Build history of the part. All positions in model axes, mm. A direction names the side the tool comes from. Round coordinates to 2 decimals unless told otherwise and drop trailing zeros. Loops run counter-clockwise (first coordinate to the right, second up) from the corner with the lowest first, then second, coordinate; pieces in that order, holes last. Notation, with made-up numbers: M 3,46.25 L 16,46.25 A15 ccw 16,55.25 Z; hole C 57,9 d3. An arc over 180 degrees is marked long. One line per item, written item: value.
```python
from build123d import *

# Parameters (mm, degrees)
SKETCH1_R                     = 4.7625
BOSS_EXTRUDE1_DEPTH           = 6.35
SKETCH7_W                     = 6.35
SKETCH7_H                     = 6.1722
BOSS_EXTRUDE2_DEPTH           = 1.016
SKETCH8_W                     = 6.35
SKETCH8_H                     = 6.1722
BOSS_EXTRUDE3_DEPTH           = 1.016
TAP_DRILL_FOR_6_32_TAP1_D     = 2.7051
TAP_DRILL_FOR_6_32_TAP1_DEPTH = 6.35
TAP_DRILL_FOR_6_32_TAP1_TIP   = 0.81269403
TAP_DRILL_FOR_6_32_TAP2_D     = 2.7051
TAP_DRILL_FOR_6_32_TAP2_DEPTH = 6.35
TAP_DRILL_FOR_6_32_TAP2_TIP   = 0.81269403
TAP_DRILL_FOR_6_32_TAP3_D     = 2.7051
TAP_DRILL_FOR_6_32_TAP3_DEPTH = 6.35
TAP_DRILL_FOR_6_32_TAP3_TIP   = 0.81269403
SKETCH18_W                    = 53.721
SKETCH18_H                    = 12.7
CUT_EXTRUDE1_DEPTH            = 3.175
FILLET1_R                     = 2.54
SKETCH19_W                    = 6.19125
SKETCH19_H                    = 31.625875518
SKETCH19_H_2                  = 31.500730808
BOSS_EXTRUDE4_DEPTH           = 3.175
CUT_EXTRUDE2_DEPTH            = 131.329786024
TAP_DRILL_FOR_6_32_TAP4_D     = 2.7051
TAP_DRILL_FOR_6_32_TAP4_DEPTH = 10.16
TAP_DRILL_FOR_6_32_TAP4_TIP   = 0.81269403
SKETCH23_W                    = 6.12775
SKETCH23_H                    = 49.2125
SKETCH23_H_2                  = 49.276
BOSS_EXTRUDE5_DEPTH           = 1.5875


with BuildPart() as part:
    # Sketch1 → Boss-Extrude1 (new body)
    with BuildSketch(Plane(origin=(0, 0, 0), x_dir=(0, 0, -1), z_dir=(1, 0, 0))):
        Polygon((0, 0), (-14.664696837, 25.4), (-112.335303163, 25.4), (-127, 0), align=None)
        with Locations((-98.298, 12.7)):
            Circle(SKETCH1_R, mode=Mode.SUBTRACT)
        with Locations((-28.702, 12.7)):
            Circle(SKETCH1_R, mode=Mode.SUBTRACT)
    extrude(amount=BOSS_EXTRUDE1_DEPTH)

    # Sketch7 → Boss-Extrude2 (add)
    with BuildSketch(Plane(origin=(0, 0, 0), x_dir=(-1, 0, 0), z_dir=(0, 0.499999999999998, -0.8660254037844397))):
        with Locations((-3.175, 19.893293675)):
            Rectangle(SKETCH7_W, SKETCH7_H)
    extrude(amount=BOSS_EXTRUDE2_DEPTH)

    # Sketch8 → Boss-Extrude3 (add)
    with BuildSketch(Plane(origin=(0, 54.99261314, 95.25), x_dir=(1, 0, 0), z_dir=(0, 0.500000000000004, 0.8660254037844365))):
        with Locations((3.175, -43.606706325)):
            Rectangle(SKETCH8_W, SKETCH8_H)
    extrude(amount=BOSS_EXTRUDE3_DEPTH)

    # Tap Drill for #6-32 Tap1
    with Locations(Plane(origin=(6.35, 0, 0), x_dir=(0, 0, -1), z_dir=(1, 0, 0))):
        with Locations((-111.761034973, 17.736097687), (-15.238965027, 17.736097687), (-119.38, 3.81), (-7.62, 3.81), (-63.5, 3.81)):
            Hole(TAP_DRILL_FOR_6_32_TAP1_D / 2, depth=TAP_DRILL_FOR_6_32_TAP1_DEPTH)
            with Locations((0, 0, -(TAP_DRILL_FOR_6_32_TAP1_DEPTH + TAP_DRILL_FOR_6_32_TAP1_TIP / 2))):  # 118° drill point
                Cone(0, TAP_DRILL_FOR_6_32_TAP1_D / 2, TAP_DRILL_FOR_6_32_TAP1_TIP, mode=Mode.SUBTRACT)

    # Tap Drill for #6-32 Tap2
    with Locations(Plane(origin=(0, 54.99261314, 95.25), x_dir=(1, 0, 0), z_dir=(0, 0.500000000000004, 0.8660254037844365))):
        with Locations((3.175, -51.633106325)):
            Hole(TAP_DRILL_FOR_6_32_TAP2_D / 2, depth=TAP_DRILL_FOR_6_32_TAP2_DEPTH)
            with Locations((0, 0, -(TAP_DRILL_FOR_6_32_TAP2_DEPTH + TAP_DRILL_FOR_6_32_TAP2_TIP / 2))):  # 118° drill point
                Cone(0, TAP_DRILL_FOR_6_32_TAP2_D / 2, TAP_DRILL_FOR_6_32_TAP2_TIP, mode=Mode.SUBTRACT)

    # Tap Drill for #6-32 Tap3
    with Locations(Plane(origin=(0, 0, 0), x_dir=(-1, 0, 0), z_dir=(0, 0.49999999999999806, -0.8660254037844398))):
        with Locations((-3.175, 11.866893675)):
            Hole(TAP_DRILL_FOR_6_32_TAP3_D / 2, depth=TAP_DRILL_FOR_6_32_TAP3_DEPTH)
            with Locations((0, 0, -(TAP_DRILL_FOR_6_32_TAP3_DEPTH + TAP_DRILL_FOR_6_32_TAP3_TIP / 2))):  # 118° drill point
                Cone(0, TAP_DRILL_FOR_6_32_TAP3_D / 2, TAP_DRILL_FOR_6_32_TAP3_TIP, mode=Mode.SUBTRACT)

    # Sketch18 → Cut-Extrude1 (cut)
    with BuildSketch(Plane.ZY):
        with Locations((63.5, 14.2875)):
            Rectangle(SKETCH18_W, SKETCH18_H)
    extrude(amount=-CUT_EXTRUDE1_DEPTH, mode=Mode.SUBTRACT)

    # Fillet1
    fillet1_edges = [part.edges().sort_by_distance(p)[0] for p in [
        (1.5875, 7.9375, 36.6395),
        (1.5875, 20.6375, 36.6395),
        (1.5875, 20.6375, 90.3605),
        (1.5875, 7.9375, 90.3605),
    ]]
    fillet(fillet1_edges, radius=FILLET1_R)

    # Sketch19 → Boss-Extrude4 (add)
    with BuildSketch(Plane(origin=(0, 25.4, 0), x_dir=(1, 0, 0), z_dir=(0, 1, 0))):
        with Locations((3.254375, -30.477634596)):
            Rectangle(SKETCH19_W, SKETCH19_H)
        with Locations((3.254375, -96.584937759)):
            Rectangle(SKETCH19_W, SKETCH19_H_2)
    extrude(amount=BOSS_EXTRUDE4_DEPTH)

    # Sketch20 → Cut-Extrude2 (cut, through all)
    with BuildSketch(Plane(origin=(6.35, 0, 0), x_dir=(0, 0, -1), z_dir=(1, 0, 0))):
        Polygon((-112.335303163, 25.4), (-110.502216058, 28.575), (-112.335303163, 28.575), align=None)
        Polygon((-14.664696837, 25.4), (-16.497783942, 28.575), (-14.664696837, 28.575), align=None)
    extrude(amount=-CUT_EXTRUDE2_DEPTH, mode=Mode.SUBTRACT)

    # Tap Drill for #6-32 Tap4
    with Locations(Plane(origin=(0, 25.4, 0), x_dir=(1, 0, 0), z_dir=(0, 1, 0))):
        with Locations((3.254375, -63.5)):
            Hole(TAP_DRILL_FOR_6_32_TAP4_D / 2, depth=TAP_DRILL_FOR_6_32_TAP4_DEPTH)
            with Locations((0, 0, -(TAP_DRILL_FOR_6_32_TAP4_DEPTH + TAP_DRILL_FOR_6_32_TAP4_TIP / 2))):  # 118° drill point
                Cone(0, TAP_DRILL_FOR_6_32_TAP4_D / 2, TAP_DRILL_FOR_6_32_TAP4_TIP, mode=Mode.SUBTRACT)

    # Sketch23 → Boss-Extrude5 (add)
    with BuildSketch(Plane.XZ):
        with Locations((3.286125, 102.39375)):
            Rectangle(SKETCH23_W, SKETCH23_H)
        with Locations((3.286125, 24.638)):
            Rectangle(SKETCH23_W, SKETCH23_H_2)
    extrude(amount=BOSS_EXTRUDE5_DEPTH)


solid = part.part
```
Item 1: Drop flat-ended pins along their axis: P1, Ø1.6, axis at x = 1.5, z = 57.5, coming from the -Y side; P2, Ø1.5, axis at x = 2, y = 14.5, coming from the +Z side; P3, Ø2.5, axis at x = 3.25, z = 63.5, coming from the +Y side. Give the stop position or say it passes through.
Check values:
P1: stops at y = 0
P2: stops at z = 119.48
P3: stops at y = 15.18
Item 2: Slice it at B-B, the plane y = 27.5. Give the cut face in (x, z).
Check values:
outline: M 0.16,15.88 L 6.35,15.88 L 6.35,46.29 L 0.16,46.29 Z; M 0.16,80.83 L 6.35,80.83 L 6.35,111.12 L 0.16,111.12 Z
Item 3: Slice it at C-C, the plane y = 12.7. Give the number of separate pieces and of enclosed holes in the cut face, and give its area (3 significant figures).
Check values:
separate pieces: 3
enclosed holes: 0
area: 422 mm2
Item 4: Slice it at D-D, the plane y = 3.81. Give the cut face in (x, z).
Check values:
outline: M 0,2.2 L 6.35,2.2 L 6.35,6.27 L 0,6.27 Z; M 0,8.97 L 6.35,8.97 L 6.35,62.15 L 0,62.15 Z; M 0,64.85 L 6.35,64.85 L 6.35,118.03 L 0,118.03 Z; M 0,120.73 L 6.35,120.73 L 6.35,124.8 L 0,124.8 Z
Item 5: Wall check: line 1 along Y through (x, z) = (1.5, 63.5); line 2 along Y through (x, z) = (2.25, 48.5); line 3 along Y through (x, z) = (3, 83) (1 decimal). Give the ranges that are in metal, low to high.
Check values:
line 1: y = 0 to 2.46, 5.16 to 7.94, 20.64 to 25.4
line 2: y = -1.59 to 7.94, 20.64 to 25.4
line 3: y = -1.6 to 7.9, 20.6 to 28.6
Item 6: Pull direction Y, two halves, no side cores. Call faces 1 (the face through (1.61, 19.91, 89.6)), 2 (the face through (2.102, 7.955, 8.31)), 3 (the face through (0.159, 27, 97)), 4 (the face through (3, -1.588, 103)): pulls with the +Y half, pulls with the -Y half, needs draft (parallel to the pull), parting line crosses it, or undercut.
Check values:
face 1: undercut
face 2: undercut
face 3: needs draft
face 4: pulls with the -Y half
Item 7: Which spindle directions (+Z, -Z, +X, -X, +Y, -Y) get a long thin tool onto all of the face, cutting with end or side? Do faces 5 (the face through (3.219, 17.774, 9.088)), 6 (the face through (3, 27, 80.835)), 7 (the face through (4.606, 21.378, 63.441)), 8 (the face through (1.6, 20.638, 63.2)). Say none if no direction does.
Check values:
face 5: -Z, +X, -X, +Y
face 6: +X, -X, +Y
face 7: +Y
face 8: -X
